Source: CAD feature listing. Evaluate the final solid. Frame: model axes, mm. A direction names the side the tool comes from. Round coordinates to 2 decimals unless told otherwise and drop trailing zeros. Loops run counter-clockwise (first coordinate to the right, second up) from the corner with the lowest first, then second, coordinate; pieces in that order, holes last. Notation, with made-up numbers: M 43.25,45.5 L 64.25,45.5 A23 ccw 64.25,56.5 Z; hole C -29.75,-7 d1. An arc over 180 degrees is marked long. Answer as CSV lines item,"result". Start each with the question number.
```python
from build123d import *

# Parameters (mm, degrees)
F0_R          = 12.5
F0_R_2        = 8
F1_DEPTH      = 75
F1_DEPTH_BACK = 75
F2_W          = 500
F2_H          = 25
F3_DEPTH      = 5
F3_DEPTH_BACK = 5
F4_R          = 8
F5_DEPTH      = 25
F5_DEPTH_BACK = 25
F6_W          = 50
F6_H          = 50
F6_W_2        = 10
F6_H_2        = 25
F7_DEPTH      = 30
F9_DEPTH      = 50
F10_W         = 12.5
F10_H         = 58.3095189485
F11_DEPTH     = 50
F12_R         = 5
F13_DEPTH     = 100.001


with BuildPart() as f1:
    # F0 (on Right) → F1 (new body, two sides)
    with BuildSketch(Plane.YZ) as f1_sk:
        Circle(F0_R)
        Circle(F0_R_2, mode=Mode.SUBTRACT)
    extrude(amount=F1_DEPTH)
    extrude(f1_sk.sketch, amount=-F1_DEPTH_BACK)

    # F2 (on Right) → F3 (join, two sides)
    with BuildSketch(Plane.YZ) as f3_sk:
        with Locations((-250, 0)):
            Rectangle(F2_W, F2_H)
    extrude(amount=F3_DEPTH)
    extrude(f3_sk.sketch, amount=-F3_DEPTH_BACK)

    # F4 (on face) → F5 (cut, two sides)
    with BuildSketch(Plane.YZ.offset(5)) as f5_sk:
        with Locations((-312.5, 0)):
            Circle(F4_R)
    extrude(amount=F5_DEPTH, mode=Mode.SUBTRACT)
    extrude(f5_sk.sketch, amount=-F5_DEPTH_BACK, mode=Mode.SUBTRACT)

    # F6 (on face) → F7 (join)
    with BuildSketch(Plane.XZ.offset(500)):
        Rectangle(F6_W, F6_H)
        Rectangle(F6_W_2, F6_H_2, mode=Mode.SUBTRACT)
        Rectangle(F6_W_2, F6_H_2)
    extrude(amount=F7_DEPTH)

    # F8 (on face) → F9 (cut)
    with BuildSketch(Plane.YZ.offset(25)):
        Polygon((-530, 25), (-530, -25), (-500, 25), align=None)
    extrude(amount=-F9_DEPTH, mode=Mode.SUBTRACT)

    # F10 (on face) → F11 (join)
    with BuildSketch(Plane(origin=(0, -378.6764705882, 227.2058823529), x_dir=(1, 0, 0), z_dir=(0, -0.8574929257, 0.5144957554))):
        with Locations((-18.75, -264.9653140452)):
            Rectangle(F10_W, F10_H)
        with Locations((18.75, -264.9653140452)):
            Rectangle(F10_W, F10_H)
    extrude(amount=F11_DEPTH)

    # F12 (on face) → F13 (cut, through all)
    with BuildSketch(Plane.YZ.offset(25)):
        with Locations((-546.9936727221, 20.5359361312)):
            Circle(F12_R)
    extrude(amount=-F13_DEPTH, mode=Mode.SUBTRACT)


solid = f1.part
```
1) Contact query for flat-ended pins moving along their axis: pin 1 Ø5 at (x, z) = (2.5, -4) entering from +Y; pin 2 Ø10 at (y, z) = (-77, 6) entering from +X; pin 3 Ø22 at (y, z) = (-550, 29) entering from -X. Output: stop coordinate, or through.
2) Section B-B, the plane y = -312.5. Return loops of the section in (x, z).
3) Section C-C, the plane x = 49.5. Return loops of the section in (y, z).
4) Mould query, pull axis Z, two halves, no side actions, for faces 5 (the flat face through (0, -515, -25)), 6 (the flat face through (-12.5, -536, 12)), 7 (the flat face through (0, 0, 0)), 8 (the flat face through (0, -253, 12.5)). Classes: pulls with the +Z half, pulls with the -Z half, needs draft (parallel to the pull), parting line crosses it, or undercut.
5) Section D-D, the plane y = -251. Return loops of the section in (x, z).
6) Section A-A, the plane x = 20. Return loops of the section in (y, z).
7) Ray query, line 1 along Z through (x, y) = (23, 0); line 2 along X through (y, z) = (-211.5, -6). Return the intervals inside material, ascending.
8) Access query for faces 1 (the flat face through (0, -253, -12.5)), 2 (the flat face through (25, -528, 12)), 3 (the flat face through (-25, -532, 10)), 4 (the cylindrical face through (1.05, 11.923, 3.755)). Directions: +Z, -Z, +X, -X, +Y, -Y. A direction counts if a zero-diameter tool reaches every point of the face in a straight line with its end or side. Return the directions, or none.
Findings below:
1,pin 1,"y = 12.41"
1,pin 2,"x = 5"
1,pin 3,"x = -25"
2,outline,"M -5,-12.5 L 5,-12.5 L 5,-8 L -5,-8 Z; M -5,8 L 5,8 L 5,12.5 L -5,12.5 Z"
3,outline,"C 0,0 d25; hole C 0,0 d16"
4,face 5,"pulls with the -Z half"
4,face 6,"needs draft"
4,face 7,"undercut"
4,face 8,"pulls with the +Z half"
5,outline,"M -5,-12.5 L 5,-12.5 L 5,12.5 L -5,12.5 Z"
6,outline,"M -572.87,0.72 L -530,-25 L -500,-25 L -500,25 L -542.87,50.72 Z; C 0,0 d25; hole C -546.99,20.54 d10; hole C 0,0 d16"
7,line 1,"-12.5 to -8, 8 to 12.5"
7,line 2,"-5 to 5"
8,face 1,"-Z, +X, -X, +Y"
8,face 2,"+Z, -Z, +X, -Y"
8,face 3,"+Z, -Z, -X, -Y"
8,face 4,"none"
